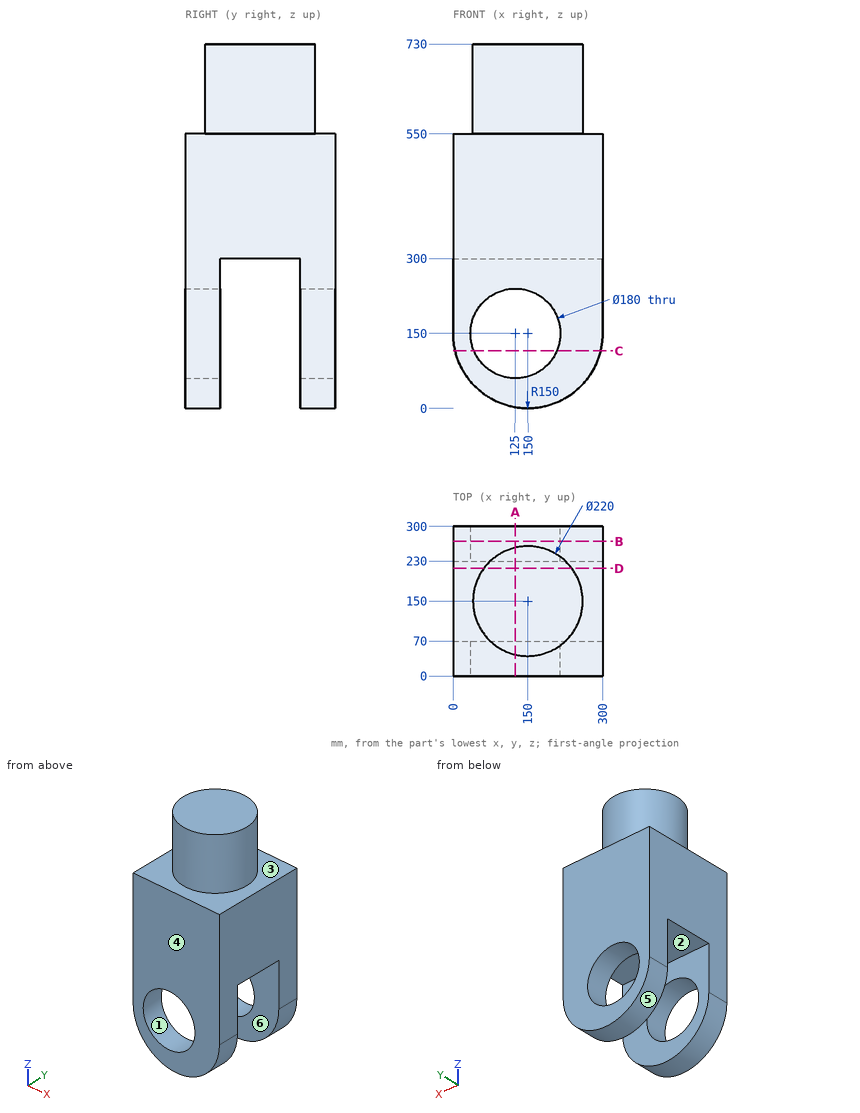
Study the drawing (mm; zero at the part's minimum x, y, z) and answer. A direction names the side the tool comes from. Coordinates: 2 decimals unless noted, no trailing zeros. Order: outer loops, then holes, each group sorted by start corner. A loop starts at its lowest first (then second) coordinate and runs counter-clockwise, first axis right, second up. Notation, with made-up numbers: (75, -26.75) -> (92, -26.75) arc R15 cw to (92, -17.75) -> close; hole circle Ø2 at (47.25, 45.25). An arc over 180 degrees is marked (long way). Answer in a Markdown table with one row per item. Add a question column.
Item 1: Find section A-A (x = 125). Write down the section's boundary in (y, z), then the cut area to 3 significant figures.
Item 2: Find section B-B (y = 270). Write down the section's boundary in (x, z), then the cut area to 3 significant figures.
Item 3: Find the intervals of material crossed by L1, parallel to Y at x = 35.5, z = 113.5; L2, parallel to Z at x = 230, y = 186; L3, parallel to Z at x = 125, y = 271, in increasing order. Write a range as from..to.
Item 4: Each of these flat-tipped pins is pushed along its axis until it touches: P1, Ø5, axis at x = 87, y = 68, coming from the -Z side; P2, Ø5, axis at x = 33.5, y = 180.5, coming from the +Z side; P3, Ø3, axis at x = 264, y = 173.5, coming from the -Z side. Where does it stop, or does it pass through?
Item 5: Find section D-D (y = 215.5). Write down the section's boundary in (x, z), then the cut area to 3 significant figures.
Item 6: Which of the six approach directions +Z, -Z, +X, -X, +Y, -Y give full straight-line access (tool end or side, diameter ignored) to the marked faces 1, 2 and 3?
Item 7: Determine the mould class of the marked faces 4, 5 and 6 for opening direction Y: +Y half, -Y half, draft (parallel to the pull), parting line (faces both ways), or undercut.
Item 8: Find section C-C (z = 115). Write down the section's boundary in (x, y), then the cut area to 3 significant figures.
Result set:
| question | item | result |
|---|---|---|
| 1 | outline | (0, 2.1) -> (70, 2.1) -> (70, 60) -> (0, 60) -> close; (0, 240) -> (70, 240) -> (70, 300) -> (230, 300) -> (230, 240) -> (300, 240) -> (300, 550) -> (257.12, 550) -> (257.12, 730) -> (42.88, 730) -> (42.88, 550) -> (0, 550) -> close; (230, 2.1) -> (300, 2.1) -> (300, 60) -> (230, 60) -> close |
| 1 | area | 130,000 mm² |
| 2 | outline | (0, 150) arc R150 ccw to (300, 150) -> (300, 550) -> (0, 550) -> close; hole circle Ø180 at (125, 150) |
| 2 | area | 130,000 mm² |
| 3 | L1 | y = 0..70, 230..300 |
| 3 | L2 | z = 300..730 |
| 3 | L3 | z = 2.1..60, 240..550 |
| 4 | P1 | stops at z = 12.74 |
| 4 | P2 | stops at z = 550 |
| 4 | P3 | stops at z = 300 |
| 5 | outline | (0, 300) -> (300, 300) -> (300, 550) -> (238.37, 550) -> (238.37, 730) -> (61.63, 730) -> (61.63, 550) -> (0, 550) -> close |
| 5 | area | 107,000 mm² |
| 6 | face 1 | +Y, -Y |
| 6 | face 2 | -Z, +X, -X |
| 6 | face 3 | +Z |
| 7 | face 4 | -Y half |
| 7 | face 5 | draft |
| 7 | face 6 | undercut |
| 8 | outline | (4.14, 0) -> (42.08, 0) -> (42.08, 70) -> (4.14, 70) -> close; (4.14, 230) -> (42.08, 230) -> (42.08, 300) -> (4.14, 300) -> close; (207.92, 0) -> (295.86, 0) -> (295.86, 70) -> (207.92, 70) -> close; (207.92, 230) -> (295.86, 230) -> (295.86, 300) -> (207.92, 300) -> close |
| 8 | area | 17,600 mm² |
